The listing builds one solid part. Answer for the finished solid, in the listing's coordinates (mm). Round coordinates to 2 decimals unless told otherwise and drop trailing zeros. Order: outer loops, then holes, each group sorted by start corner. A loop starts at its lowest first (then second) coordinate and runs counter-clockwise, first axis right, second up. Notation, with made-up numbers: M -25,-5 L 18,-5 A22 ccw 18,6 Z; hole C -22.75,-28 d6. An arc over 180 degrees is marked long. Put each result on its own line as item: value. Start each with the question number.
1. The part is cut by section A-A (x = 141). Give the vertices of the cut face in (y, z), then the cut area to 3 significant figures.
2. The part is cut by section C-C (z = 48). Give the vertices of the cut face in (x, y).
3. The mould has two halves that part along Z. Classify faces 1 (the face through (38, 5, 67.407)), 2 (the face through (-50.11, 5.07, -14.29)), 3 (the face through (-180.253, 4.93, -38.745)), 4 (the face through (149.89, 5.07, -14.29)): +Z half, -Z half, draft (parallel to the pull), parting line (faces both ways), or undercut.
4. The part is cut by section D-D (x = 212). Give the vertices of the cut face in (y, z), then the cut area to 3 significant figures.
5. Consider line 1 (X direction, y = 2, z = -22); line 2 (X direction, y = 9, z = -3); line 3 (X direction, y = 3.75, z = 18). Determine where each line is inside the solid, lowest interval first.
6. Each of these flat-tipped pins is pushed along its axis until it touches: pin 1 Ø21 at (x, z) = (137, -12.59) entering from +Y; pin 2 Ø1.5 at (y, z) = (6.5, 15.5) entering from -X. Where does it stop, or does it pass through?
7. The part is cut by section B-B (y = 2). Give the vertices of the cut face in (x, z).
from build123d import *

# Parameters (mm, degrees)
BOSS_EXTRUDE1_DEPTH = 10
SKETCH2_R           = 13
CUT_EXTRUDE1_DEPTH  = 10
CUT_EXTRUDE2_DEPTH  = 10


with BuildPart() as part:
    # Sketch1 → Boss-Extrude1 (new body)
    with BuildSketch(Plane(origin=(0, 0, 0), x_dir=(1, 0, 0), z_dir=(0, 1, 0))):
        with BuildLine():
            Line((248.032931618, 52.593341059), (260.305567907, 25.2785247))
            ThreePointArc((260.305567907, 25.2785247), (260.612237386, 17.847313664), (255.703480887, 12.259733394))
            Line((255.703480887, 12.259733394), (41.520626689, -96.255259938))
            ThreePointArc((41.520626689, -96.255259938), (37.001121909, -97.334829649), (32.481617129, -96.255259938))
            Line((32.481617129, -96.255259938), (-181.70123707, 12.259733394))
            ThreePointArc((-181.70123707, 12.259733394), (-186.609993569, 17.847313664), (-186.30332409, 25.2785247))
            Line((-186.30332409, 25.2785247), (-174.0306878, 52.593341059))
            Line((-174.0306878, 52.593341059), (248.032931618, 52.593341059))
        make_face()
    extrude(amount=BOSS_EXTRUDE1_DEPTH)

    # Sketch2 → Cut-Extrude1 (cut)
    with BuildSketch(Plane(origin=(0, 10, 0), x_dir=(1, 0, 0), z_dir=(0, 1, 0))):
        with Locations(Location((137.001121909, 12.593341059, 0), (0, 0, 270))):
            Circle(SKETCH2_R)
        with Locations(Location((-62.998878091, 12.593341059, 0), (0, 0, 270))):
            Circle(SKETCH2_R)
    extrude(amount=-CUT_EXTRUDE1_DEPTH, mode=Mode.SUBTRACT)

    # Sketch3 → Cut-Extrude2 (cut)
    with BuildSketch(Plane(origin=(0, 10, 0), x_dir=(1, 0, 0), z_dir=(0, 1, 0))):
        Polygon((37.001121909, -67.406658941), (125.459060888, -67.406658941), (125.459060888, -160.473444946), (-80.94279673, -160.473444946), (-80.94279673, -67.406658941), align=None)
    extrude(amount=-CUT_EXTRUDE2_DEPTH, mode=Mode.SUBTRACT)


solid = part.part
Resolved:
1. outline: M 0,-52.59 L 10,-52.59 L 10,-24.96 L 0,-24.96 Z; M 0,-0.22 L 10,-0.22 L 10,45.85 L 0,45.85 Z
1. area: 737 mm2
2. outline: M -62.76,0 L 136.77,0 L 136.77,10 L -62.76,10 Z
3. face 1: +Z half
3. face 2: undercut
3. face 3: -Z half
3. face 4: undercut
4. outline: M 0,-52.59 L 10,-52.59 L 10,9.88 L 0,9.88 Z
4. area: 625 mm2
5. line 1: -187.15 to -71.97, -54.03 to 128.03, 145.97 to 261.15
5. line 2: -163.42 to -71.77, -54.23 to 128.23, 145.77 to 237.43
5. line 3: -121.98 to 195.98
6. pin 1: through
6. pin 2: x = -128.39
7. outline: M -186.3,-25.28 L -174.03,-52.59 L 248.03,-52.59 L 260.31,-25.28 A10 ccw 255.7,-12.26 L 98.46,67.41 L -24.46,67.41 L -181.7,-12.26 A10 ccw Z; hole C -63,-12.59 d26; hole C 137,-12.59 d26
